```python
from build123d import *

# Parameters (mm, degrees)
SKETCH1_W           = 14
SKETCH1_H           = 8
BOSS_EXTRUDE1_DEPTH = 8
SKETCH3_R           = 2.15
BOSS_EXTRUDE3_DEPTH = 4.5
BOSS_EXTRUDE4_START = 4.5
SKETCH4_R           = 2.15
BOSS_EXTRUDE4_DEPTH = 4.5


with BuildPart() as part:
    # Sketch1 → Boss-Extrude1 (new body)
    with BuildSketch(Plane(origin=(0, 0, 0), x_dir=(1, 0, 0), z_dir=(0, 1, 0))):
        with Locations((17.805194805, 5.675324675)):
            Rectangle(SKETCH1_W, SKETCH1_H)
    extrude(amount=BOSS_EXTRUDE1_DEPTH)

    # Sketch3 → Boss-Extrude3 (add)
    with BuildSketch(Plane(origin=(24.805194805, 0, 0), x_dir=(0, 0, -1), z_dir=(1, 0, 0))):
        with Locations(Location((5.675324675, 4, 0), (0, 0, 180))):
            Circle(SKETCH3_R)
    extrude(amount=BOSS_EXTRUDE3_DEPTH)

    # Sketch4 → Boss-Extrude4 (add)
    with BuildSketch(Plane.ZY.offset(-10.805194805).offset(BOSS_EXTRUDE4_START)):
        with Locations((-5.675324675, 4)):
            Circle(SKETCH4_R)
    extrude(amount=-BOSS_EXTRUDE4_DEPTH)


solid = part.part
```
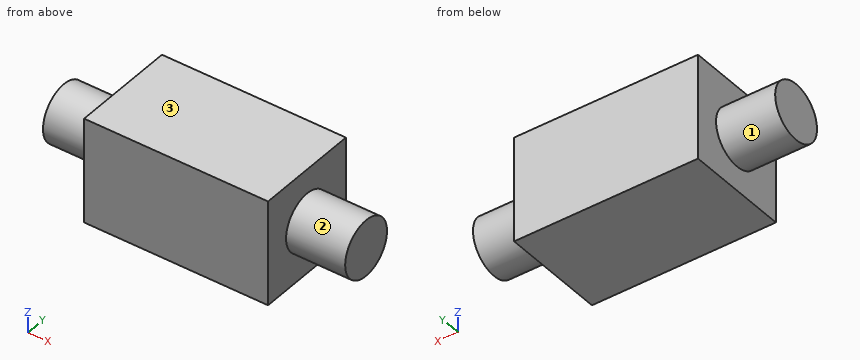
CAD build for the part. Positions are in the model's coordinates, mm. Face numbers are marked on the shaded views. A direction names the side the tool comes from. Coordinates: 2 decimals unless noted, no trailing zeros. Write each loop counter-clockwise with the first axis right and the second up, starting at its lowest first coordinate (ties: lowest second). Pieces come first, ordered by that corner, then holes.
(1) Cut at A-A, the plane y = 4. List the corners of the cut face in (x, z).
(2) Cut at B-B, the plane z = -4. List the corners of the cut face in (x, y), and give its area (3 significant figures).
(3) 3-axis set-ups, long thin cutter, end or side, ignore diameter. For the marked faces 1, 2 and 3: which of +Z, -Z, +X, -X, +Y, -Y reach the whole face in a straight line?
(4) Cut at C-C, the plane x = 27.75. List the corners of the cut face in (y, z), and give its area (3 significant figures).
(5) Drill centre lines: probe 1 along X at (y, z) = (0.5, -5.5); probe 2 along Y at (x, z) = (8.25, -4.5); probe 3 along Z at (x, y) = (28, 5.75). Where is each one in solid material? Low to high.
(6) Cut at D-D, the plane z = -2.5. List the corners of the cut face in (x, y), and give its area (3 significant figures).
Geometry says:
1. outline: (6.31, -7.83) - (10.81, -7.83) - (10.81, -9.68) - (24.81, -9.68) - (24.81, -7.83) - (29.31, -7.83) - (29.31, -3.53) - (24.81, -3.53) - (24.81, -1.68) - (10.81, -1.68) - (10.81, -3.53) - (6.31, -3.53) - close
2. outline: (6.31, 2.65) - (10.81, 2.65) - (10.81, 0) - (24.81, 0) - (24.81, 2.65) - (29.31, 2.65) - (29.31, 5.35) - (24.81, 5.35) - (24.81, 8) - (10.81, 8) - (10.81, 5.35) - (6.31, 5.35) - close
2. area: 136 mm2
3. face 1: -X
3. face 2: +X
3. face 3: +Z, +X, -X, +Y, -Y
4. outline: circle Ø4.3 at (4, -5.68)
4. area: 14.5 mm2
5. probe 1: x = 10.81 to 24.81
5. probe 2: y = 2.2 to 5.8
5. probe 3: z = -6.92 to -4.43
6. outline: (10.81, 0) - (24.81, 0) - (24.81, 8) - (10.81, 8) - close
6. area: 112 mm2
